from build123d import *

# Parameters (mm, degrees)
SKETCH2_W           = 100.076
SKETCH2_H           = 100.076
BOSS_EXTRUDE2_DEPTH = 12.7
FILLET1_R           = 19.05
SKETCH3_W           = 4.948209201
SKETCH3_H           = 46.039859528
CUT_EXTRUDE1_DEPTH  = 9.906


with BuildPart() as part:
    # Sketch2 → Boss-Extrude2 (new body)
    with BuildSketch(Plane.XY):
        with Locations((20.865266409, -15.842146718)):
            Rectangle(SKETCH2_W, SKETCH2_H)
    extrude(amount=BOSS_EXTRUDE2_DEPTH)

    # Fillet1
    fillet1_edges = [part.edges().sort_by_distance(p)[0] for p in [
        (-29.172733591, 34.195853282, 6.35),
        (70.903266409, 34.195853282, 6.35),
        (70.903266409, -65.880146718, 6.35),
        (-29.172733591, -65.880146718, 6.35),
    ]]
    fillet(fillet1_edges, radius=FILLET1_R)

    # Sketch3 → Cut-Extrude1 (cut)
    with BuildSketch(Plane(origin=(70.903266409, 0, 0), x_dir=(0, 0, -1), z_dir=(1, 0, 0))):
        with Locations((-4.90705885, -17.455693197)):
            Rectangle(SKETCH3_W, SKETCH3_H)
    extrude(amount=-CUT_EXTRUDE1_DEPTH, mode=Mode.SUBTRACT)


solid = part.part
For this review, take the finished solid that the model builds, in its own axes (mm). A direction names the side the tool comes from. Round coordinates to 2 decimals unless told otherwise and drop trailing zeros. Write each loop counter-clockwise with the first axis right and the second up, starting at its lowest first coordinate (ties: lowest second). Pieces come first, ordered by that corner, then holes. Notation, with made-up numbers: (19, 60.5) - (58, 60.5) arc R35 cw to (58, 96.5) - close; hole circle Ø11 at (79, 54.25). An arc over 180 degrees is marked (long way). Write item = value, one per line. Start each with the question number.
1. Draft analysis for pull direction Z (two halves, no side actions). For faces 3 (the face through (20, -15, 12.7)), 4 (the face through (66, -18, 2.433)), 5 (the face through (65.17, -60.45, 6.44)), state which applies: released by +Z, released by -Z, zero draft, split by the parting line, or undercut.
2. Consider section A-A on z = 5.25. State the section outline as (x, y) points, plus the area to 3 significant figures.
3. Consider section C-C on x = 59. State the section outline as (y, z) points, plus the area to 3 significant figures.
4. For faces 1 (the face through (60.997, -17, 5)), 2 (the face through (-23.74, -60.15, 6.44)), list the 3-axis set-ups (+Z, -Z, +X, -X, +Y, -Y) from which the entire face can be reached by the end or side of a thin tool; tool diameter is ignored.
5. Wall thickness on L1, parallel to Z at x = 65, y = -5.5; L2, parallel to X at y = -30, z = 6; L3, parallel to Y at x = 66.5, z = 2.5: over which ranges is each line inside the solid? List them lowest first.
6. For pin 1 Ø5.5 at (x, z) = (65.5, 4.5) entering from -Y; pin 2 Ø2.5 at (x, z) = (68.5, 4) entering from +Y, all flat-tipped, find the tip position at first contact; note any pin that passes through.
7. Consider section D-D on x = -19.5. State the section outline as (y, z) points, plus the area to 3 significant figures.
8. Consider section B-B on y = -30. State the section outline as (x, z) points, plus the area to 3 significant figures.
Evaluation:
q1.face_3 = released by +Z
q1.face_4 = undercut
q1.face_5 = zero draft
q2.outline = (-29.17, -46.83) arc R19.05 ccw to (-10.12, -65.88) - (51.85, -65.88) arc R19.05 ccw to (70.9, -46.83) - (70.9, -40.48) - (61, -40.48) - (61, 5.56) - (70.9, 5.56) - (70.9, 15.15) arc R19.05 ccw to (51.85, 34.2) - (-10.12, 34.2) arc R19.05 ccw to (-29.17, 15.15) - close
q2.area = 9,250 mm2
q3.outline = (-64.49, 0) - (32.8, 0) - (32.8, 12.7) - (-64.49, 12.7) - close
q3.area = 1,240 mm2
q4.face_1 = +X
q4.face_2 = +Z, -Z, -X, -Y
q5.L1 = 0 to 2.43, 7.38 to 12.7
q5.L2 = -29.17 to 61
q5.L3 = -59.01 to -40.48, 5.56 to 27.33
q6.pin_1 = -62.46
q6.pin_2 = 26.36
q7.outline = (-63.41, 0) - (31.73, 0) - (31.73, 12.7) - (-63.41, 12.7) - close
q7.area = 1,210 mm2
q8.outline = (-29.17, 0) - (70.9, 0) - (70.9, 2.43) - (61, 2.43) - (61, 7.38) - (70.9, 7.38) - (70.9, 12.7) - (-29.17, 12.7) - close
q8.area = 1,220 mm2
